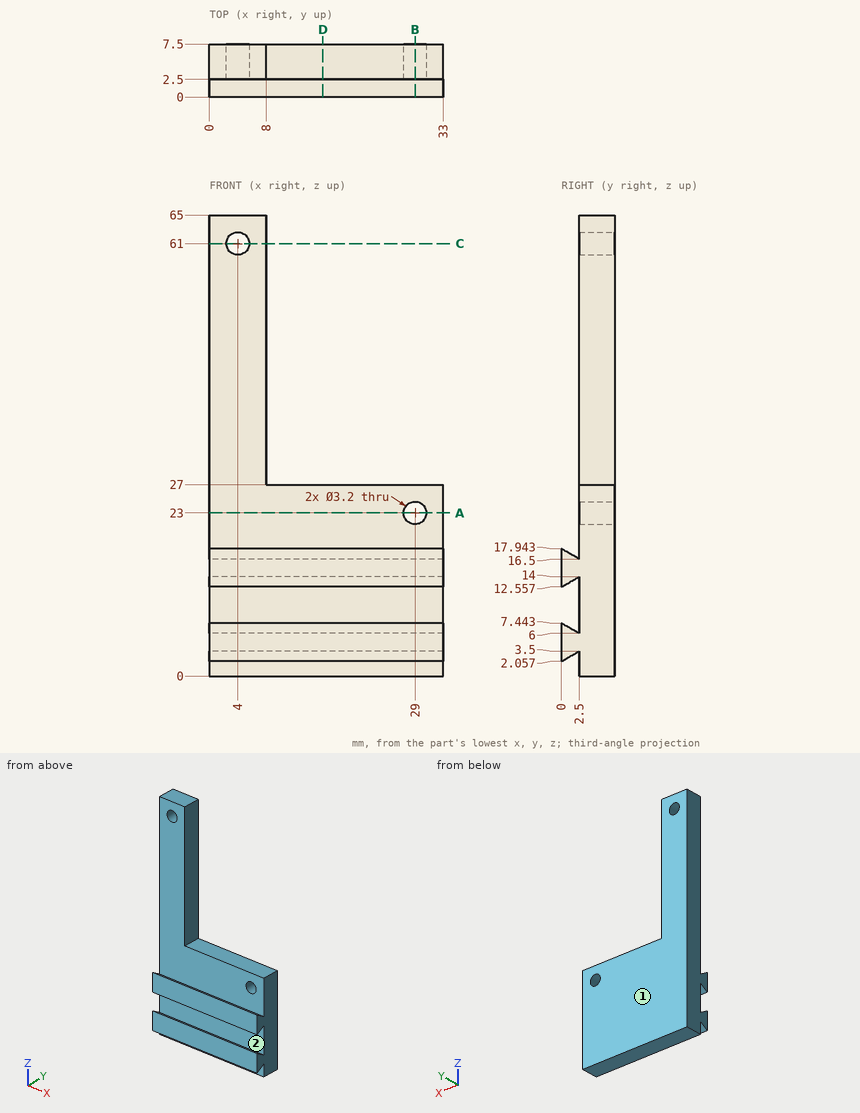
Check sheet for the drawn part. Datum: minimum x, y, z corner. Units: mm. Give positions to 0.01 mm unless a question says otherwise; leave off trailing zeros. Loops run counter-clockwise (first coordinate to the right, second up) from the corner with the lowest first, then second, coordinate; pieces in that order, holes last.
1) Thickness scan on line 1 along X through (y, z) = (4.2, 61); line 2 along X through (y, z) = (5.95, 23); line 3 along Z through (x, y) = (4, 4). Record the ranges inside material, lowest first.
2) Draft check along Z on the marked faces 1 and 2. Enter one of: pulls with the +Z half, pulls with the -Z half, needs draft (parallel to the pull), parting line crosses it, or undercut.
3) Sectioned sample at C-C, the plane z = 61. Enter the section's corners in (x, y).
4) Sectioned sample at A-A, the plane z = 23. Enter the section's corners in (x, y), then the cut area to 3 significant figures.
5) Depth check by flat-ended pin: pin 1 Ø1.9 at (x, z) = (29, 23) entering from -Y; pin 2 Ø12 at (x, z) = (13, 47) entering from -Y; pin 3 Ø2.5 at (y, z) = (5.5, 54.5) entering from +X. Enter the tip coordinate at first touch or a pass-through.
6) Sectioned sample at D-D, the plane x = 16. Enter the section's corners in (y, z).
7) Sectioned sample at B-B, the plane x = 29. Enter the section's corners in (y, z).
Answers:
1. line 1: x = 0 to 2.4, 5.6 to 8
1. line 2: x = 0 to 27.4, 30.6 to 33
1. line 3: z = 0 to 59.4, 62.6 to 65
2. face 1: needs draft
2. face 2: undercut
3. outline: (0, 2.5) - (2.4, 2.5) - (2.4, 7.5) - (0, 7.5) - close; (5.6, 2.5) - (8, 2.5) - (8, 7.5) - (5.6, 7.5) - close
4. outline: (0, 2.5) - (27.4, 2.5) - (27.4, 7.5) - (0, 7.5) - close; (30.6, 2.5) - (33, 2.5) - (33, 7.5) - (30.6, 7.5) - close
4. area: 149 mm2
5. pin 1: passes through
5. pin 2: stops at y = 2.5
5. pin 3: stops at x = 8
6. outline: (0, 2.06) - (2.5, 3.5) - (2.5, 0) - (7.5, 0) - (7.5, 27) - (2.5, 27) - (2.5, 16.5) - (0, 17.94) - (0, 12.56) - (2.5, 14) - (2.5, 6) - (0, 7.44) - close
7. outline: (0, 2.06) - (2.5, 3.5) - (2.5, 0) - (7.5, 0) - (7.5, 21.4) - (2.5, 21.4) - (2.5, 16.5) - (0, 17.94) - (0, 12.56) - (2.5, 14) - (2.5, 6) - (0, 7.44) - close; (2.5, 24.6) - (7.5, 24.6) - (7.5, 27) - (2.5, 27) - close
